```python
from build123d import *

# Parameters (mm, degrees)
F0_R     = 3.410519
F1_DEPTH = 7


with BuildPart() as f1:
    # F0 (on Top) → F1 (new body)
    with BuildSketch(Plane.XY):
        with BuildLine():
            ThreePointArc((-11.15, 0), (-5.575, 9.656183), (5.575, 9.656183))
            ThreePointArc((5.575, 9.656183), (5.339004, 11.938072), (4.641006, 14.123366))
            ThreePointArc((4.641006, 14.123366), (-11.15, 19.312367), (-14.551697, 3.042454))
            ThreePointArc((-14.551697, 3.042454), (-13.008176, 1.345323), (-11.15, 0))
        make_face()
        with Locations((-8.123896, 14.071)):
            Circle(F0_R, mode=Mode.SUBTRACT)
        with BuildLine():
            ThreePointArc((-14.551697, -3.042454), (-13.008176, -1.345323), (-11.15, 0))
            ThreePointArc((-11.15, 0), (-13.008176, 1.345323), (-14.551697, 3.042454))
            ThreePointArc((-14.551697, 3.042454), (-14.866351, 0), (-14.551697, -3.042454))
        make_face()
        with BuildLine():
            ThreePointArc((4.641006, -14.123366), (5.339004, -11.938072), (5.575, -9.656183))
            ThreePointArc((5.575, -9.656183), (-5.575, -9.656183), (-11.15, 0))
            ThreePointArc((-11.15, 0), (-13.008176, -1.345323), (-14.551697, -3.042454))
            ThreePointArc((-14.551697, -3.042454), (-11.15, -19.312367), (4.641006, -14.123366))
        make_face()
        with Locations((-8.123896, -14.071)):
            Circle(F0_R, mode=Mode.SUBTRACT)
        with BuildLine():
            ThreePointArc((9.91069, -11.080912), (7.669172, -10.592749), (5.575, -9.656183))
            ThreePointArc((5.575, -9.656183), (5.339004, -11.938072), (4.641006, -14.123366))
            ThreePointArc((4.641006, -14.123366), (7.433176, -12.874638), (9.91069, -11.080912))
        make_face()
        with BuildLine():
            ThreePointArc((5.575, 9.656183), (9.656183, 5.575), (11.15, 0))
            ThreePointArc((11.15, 0), (9.656183, -5.575), (5.575, -9.656183))
            ThreePointArc((5.575, -9.656183), (7.669172, -10.592749), (9.91069, -11.080912))
            ThreePointArc((9.91069, -11.080912), (22.3, 0), (9.91069, 11.080912))
            ThreePointArc((9.91069, 11.080912), (7.669172, 10.592749), (5.575, 9.656183))
        make_face()
        with Locations((16.247792, 0)):
            Circle(F0_R, mode=Mode.SUBTRACT)
        with BuildLine():
            ThreePointArc((4.641006, 14.123366), (5.339004, 11.938072), (5.575, 9.656183))
            ThreePointArc((5.575, 9.656183), (7.669172, 10.592749), (9.91069, 11.080912))
            ThreePointArc((9.91069, 11.080912), (7.433176, 12.874638), (4.641006, 14.123366))
        make_face()
    extrude(amount=F1_DEPTH)


solid = f1.part
```
Can you work these out from the model? Positions are in its coordinate system, mm. Coordinates: 2 decimals unless noted, no trailing zeros. Loops run counter-clockwise (first coordinate to the right, second up) from the corner with the lowest first, then second, coordinate; pieces in that order, holes last. Notation, with made-up numbers: (-26, 49) -> (0, 49) arc R19 cw to (0, 56) -> close; hole circle Ø11 at (-36, 20.5). An arc over 180 degrees is marked (long way). Put each result on its own line as item: value. Start each with the question number.
Q1. I'm going to push flat-ended pins straight in: P1, Ø3, axis at y = -16.5, z = 2.5, coming from the +X side; P2, Ø4, axis at x = 2, z = 4, coming from the +Y side; P3, Ø3, axis at y = -13.5, z = 3.5, coming from the -X side; P4, Ø2, axis at x = 17.5, y = -0.5, coming from the -Z side. Where does each tip first touch, or does it pass through?
Q2. I want a section at B-B (y = -4). Write out the boundary of the cut face in (x, z).
Q3. I want a section at C-C (z = 4.75). Write out the boundary of the cut face in (x, y) (3 decimals).
Q4. Thinking about a two-plate mould opening in X: for faces 1 (the face through (-6, 10, 0)), 2 (the face through (-10.638, 16.376, 3.451)), 3 (the face through (-11.376, -19.178, 3.451)), which applies, pulls with the +X half, pulls with the -X half, needs draft (parallel to the pull), parting line crosses it, or undercut?
Q5. I want a section at D-D (x = -12). Write out the boundary of the cut face in (y, z), plus the area to 3 significant figures.
Q6. If I drill on line 1 (Y direction, x = -5.5, z = 2.5); line 2 (Y direction, x = -7, z = 1); line 3 (Y direction, x = 8.5, z = 5.25), over which ranges is the centre line in solid material (lowest first)? Write a range as [from, to].
Q7. I want a section at A-A (x = 2.5). Write out the boundary of the cut face in (y, z).
Taken from the geometry:
1. P1: stops at x = 4.21
1. P2: stops at y = 19.31
1. P3: stops at x = -16.48
1. P4: passes through
2. outline: (-15.18, 0) -> (-10.41, 0) -> (-10.41, 7) -> (-15.18, 7) -> close; (10.41, 0) -> (21.56, 0) -> (21.56, 7) -> (10.41, 7) -> close
3. outline: (-14.552, -3.042) arc R11.15 ccw (long way) to (4.641, -14.123) arc R14.866 ccw to (9.911, -11.081) arc R11.15 ccw (long way) to (9.911, 11.081) arc R14.866 ccw to (4.641, 14.123) arc R11.15 ccw (long way) to (-14.552, 3.042) arc R14.866 ccw to start; hole circle Ø6.821 at (-8.124, -14.071); hole circle Ø6.821 at (-8.124, 14.071); hole (5.575, 9.656) arc R11.15 ccw (long way) to (11.15, 0) arc R11.15 ccw to start; hole circle Ø6.821 at (16.248, 0)
4. face 1: needs draft
4. face 2: undercut
4. face 3: parting line crosses it
5. outline: (-18.77, 0) -> (18.77, 0) -> (18.77, 7) -> (-18.77, 7) -> close
5. area: 263 mm2
6. line 1: y = [-20.81, -16.25], [-11.89, -9.7], [9.7, 11.89], [16.25, 20.81]
6. line 2: y = [-20.71, -17.29], [-10.85, -8.68], [8.68, 10.85], [17.29, 20.71]
6. line 3: y = [-12.2, -7.22], [7.22, 12.2]
7. outline: (-17.34, 0) -> (-10.87, 0) -> (-10.87, 7) -> (-17.34, 7) -> close; (10.87, 0) -> (17.34, 0) -> (17.34, 7) -> (10.87, 7) -> close
